```python
from build123d import *

# Parameters (mm, degrees)
BOSS_EXTRUDE1_DEPTH = 3.175
SKETCH2_R           = 12.5
BOSS_EXTRUDE2_DEPTH = 6.35
FILLET1_R           = 1.5875


with BuildPart() as part:
    # Sketch1 → Boss-Extrude1 (new body, symmetric)
    with BuildSketch(Plane(origin=(0, 0, 0), x_dir=(0, 0, -1), z_dir=(1, 0, 0))):
        with BuildLine():
            Line((12.5, 0), (12.5, -55.612498595))
            ThreePointArc((12.5, -55.612498595), (8.769459923, -56.321368704), (5, -56.780278266))
            Line((5, -56.780278266), (5, -50))
            ThreePointArc((5, -50), (0, -45), (-5, -50))
            Line((-5, -50), (-5, -56.780278266))
            ThreePointArc((-5, -56.780278266), (-8.769459923, -56.321368704), (-12.5, -55.612498595))
            Line((-12.5, -55.612498595), (-12.5, 0))
            ThreePointArc((-12.5, 0), (0, 12.5), (12.5, 0))
        make_face()
        with BuildLine():
            Line((-3.2004, 5.51390651), (-3.2004, -5.51390651))
            ThreePointArc((-3.2004, -5.51390651), (0, -6.3754), (3.2004, -5.51390651))
            Line((3.2004, -5.51390651), (3.2004, 5.51390651))
            ThreePointArc((3.2004, 5.51390651), (0, 6.3754), (-3.2004, 5.51390651))
        make_face(mode=Mode.SUBTRACT)
    extrude(amount=BOSS_EXTRUDE1_DEPTH, both=True)

    # Sketch2 → Boss-Extrude2 (add)
    with BuildSketch(Plane(origin=(3.175, 0, 0), x_dir=(0, 0, -1), z_dir=(1, 0, 0))):
        Circle(SKETCH2_R)
        with BuildLine():
            Line((-3.2004, 5.51390651), (-3.2004, -5.51390651))
            ThreePointArc((-3.2004, -5.51390651), (0, -6.3754), (3.2004, -5.51390651))
            Line((3.2004, -5.51390651), (3.2004, 5.51390651))
            ThreePointArc((3.2004, 5.51390651), (0, 6.3754), (-3.2004, 5.51390651))
        make_face(mode=Mode.SUBTRACT)
    extrude(amount=BOSS_EXTRUDE2_DEPTH)

    # Fillet1
    fillet1_edges = [part.edges().sort_by_distance(p)[0] for p in [
        (0, 5.51390651, -3.2004),
        (0, 5.51390651, 3.2004),
        (0, -5.51390651, 3.2004),
        (0, -5.51390651, -3.2004),
    ]]
    fillet(fillet1_edges, radius=FILLET1_R)


solid = part.part
```
The model under review builds one solid part; all positions refer to its coordinate system, in mm. A direction names the side the tool comes from. Give positions to 0.01 mm unless a question says otherwise; leave off trailing zeros. Write each loop counter-clockwise with the first axis right and the second up, starting at its lowest first coordinate (ties: lowest second). Pieces come first, ordered by that corner, then holes. Notation, with made-up numbers: (60, -11.75) -> (86, -11.75) arc R18 ccw to (86, 0.25) -> close; hole circle Ø6 at (80.5, 24). An arc over 180 degrees is marked (long way). Answer in a Markdown table with one row per item.
1) Add section C-C on y = -46. State the section outline as (x, z) points (3 decimals), plus the area to 3 significant figures.
Worked answers:
| item | result |
|---|---|
| outline | (-3.175, -12.5) -> (3.175, -12.5) -> (3.175, -3) -> (-3.175, -3) -> close; (-3.175, 3) -> (3.175, 3) -> (3.175, 12.5) -> (-3.175, 12.5) -> close |
| area | 121 mm² |
2) Clearance check with flat-ended pins moving along their axes: P1, Ø6, axis at x = 8, z = -9, coming from the -Y side; P2, Ø4, axis at x = 3, z = 7.5, coming from the -Y side; P3, Ø1, axis at x = 5.5, z = 1.5, coming from the -Y side. State where each tip first meets the part, or that it passes through.
Worked answers:
| item | result |
|---|---|
| P1 | y = -10.97 |
| P2 | y = -56.73 |
| P3 | y = -12.46 |
3) Add section D-D on x = 0.75. State the section outline as (y, z) points (1 decimal).
Worked answers:
| item | result |
|---|---|
| outline | (-56.8, -5) arc R57 ccw to (-55.6, -12.5) -> (0, -12.5) arc R12.5 ccw to (0, 12.5) -> (-55.6, 12.5) arc R57 ccw to (-56.8, 5) -> (-50, 5) arc R5 cw to (-50, -5) -> close; hole (-6, -2.1) arc R1.6 ccw to (-4.5, -3.2) -> (4.5, -3.2) arc R1.6 ccw to (6, -2.1) arc R6.4 ccw to (6, 2.1) arc R1.6 ccw to (4.5, 3.2) -> (-4.5, 3.2) arc R1.6 ccw to (-6, 2.1) arc R6.4 ccw to start |
4) For L1, parallel to Z at x = 0.5, y = -51; L2, parallel to X at y = -31, z = -6.25 (3 decimals); L3, parallel to Y at x = -2, z = -2, list the stretches that pass through material, from the lowest coordinate up. Write a range as [from, to].
Worked answers:
| item | result |
|---|---|
| L1 | [-12.5, -5], [5, 12.5] |
| L2 | [-3.175, 3.175] |
| L3 | [-45.42, -6.05], [6.05, 12.34] |
5) Tool access review of faces 1 (the flat face through (0, -53, -5)), 2 (the cylindrical face through (3.086, 6.375, -0.031)), 3 (the flat face through (9.525, 0, -5)): name each direction out of +Z, -Z, +X, -X, +Y, -Y from which nothing blocks a thin tool from reaching the whole face with its end or side.
Worked answers:
| item | result |
|---|---|
| face 1 | +X, -X, -Y |
| face 2 | +X, -X |
| face 3 | +Z, -Z, +X, +Y, -Y |
6) Add section B-B on x = 5.5. State the section outline as (y, z) points (1 decimal), plus the area to 3 significant figures.
Worked answers:
| item | result |
|---|---|
| outline | circle Ø25 at (0, 0); hole (-6, -2.1) arc R1.6 ccw to (-4.5, -3.2) -> (4.5, -3.2) arc R1.6 ccw to (6, -2.1) arc R6.4 ccw to (6, 2.1) arc R1.6 ccw to (4.5, 3.2) -> (-4.5, 3.2) arc R1.6 ccw to (-6, 2.1) arc R6.4 ccw to start |
| area | 414 mm² |
7) Add section A-A on z = 0. State the section outline as (x, y) points (3 decimals), plus the area to 3 significant figures.
Worked answers:
| item | result |
|---|---|
| outline | (-3.175, -45) -> (3.175, -45) -> (3.175, -12.5) -> (9.525, -12.5) -> (9.525, -6.375) -> (-3.175, -6.375) -> close; (-3.175, 6.375) -> (9.525, 6.375) -> (9.525, 12.5) -> (-3.175, 12.5) -> close |
| area | 362 mm² |
8) Mouldability with a two-part tool opening along Y and no side actions: class faces 4 (the cylindrical face through (0.044, -56.313, -8.822)), 5 (the cylindrical face through (3.086, 5.433, 2.903)), 6 (the flat face through (0, -53, 5)) as +Y half, -Y half, draft (parallel to the pull), parting line (faces both ways), or undercut.
Worked answers:
| item | result |
|---|---|
| face 4 | -Y half |
| face 5 | undercut |
| face 6 | draft |
